Source: three-view drawing plus pictorial views. Frame: mm from the lowest corner of the part. A direction names the side the tool comes from. Give positions to 0.01 mm unless a question says otherwise; leave off trailing zeros. Loops run counter-clockwise (first coordinate to the right, second up) from the corner with the lowest first, then second, coordinate; pieces in that order, holes last. Notation, with made-up numbers: (89, 76) - (122, 76) arc R17 ccw to (122, 108) - close; hole circle Ø9 at (8, 51.25). An arc over 180 degrees is marked (long way). Put each result on its own line as item: value.
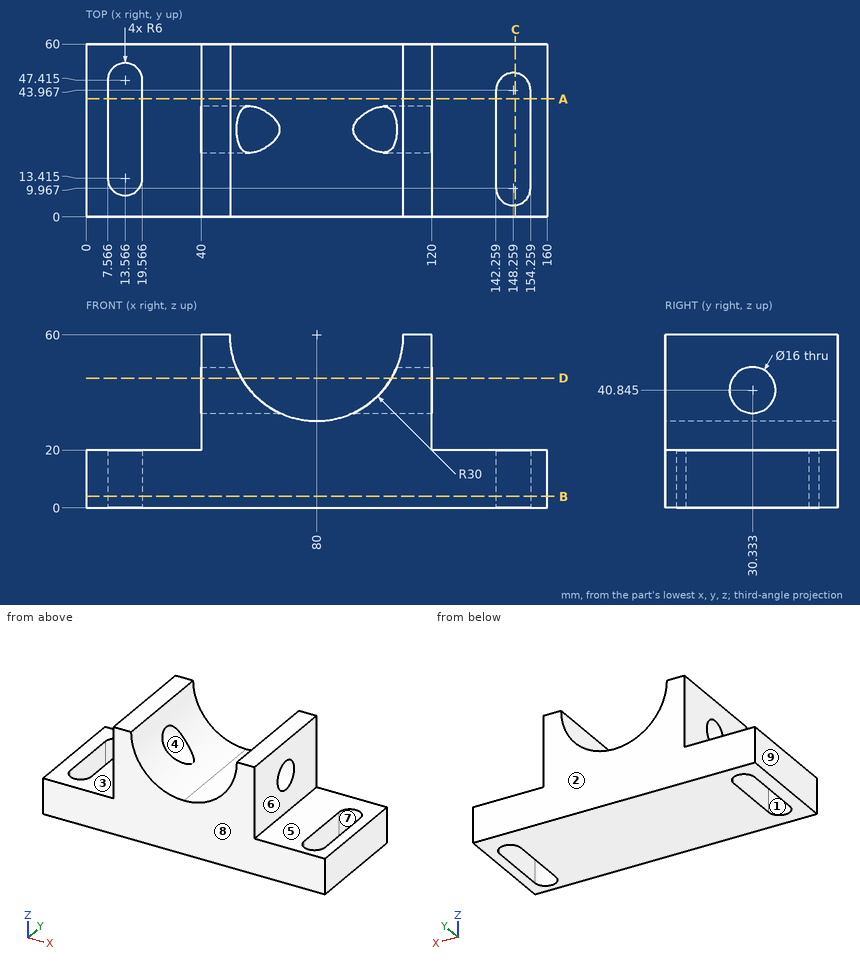
1) Section query C-C, the plane x = 149. Output: boundary loops of the cut face in (y, z), plus the area to 3 significant figures.
Check result:
outline: (0, 0) - (4.01, 0) - (4.01, 20) - (0, 20) - close; (49.92, 0) - (60, 0) - (60, 20) - (49.92, 20) - close
area: 282 mm²
2) Section query D-D, the plane z = 45. Output: boundary loops of the cut face in (x, y).
Check result:
outline: (40, 0) - (54.02, 0) - (54.02, 23.5) - (40, 23.5) - close; (40, 37.17) - (54.02, 37.17) - (54.02, 60) - (40, 60) - close; (105.98, 0) - (120, 0) - (120, 23.5) - (105.98, 23.5) - close; (105.98, 37.17) - (120, 37.17) - (120, 60) - (105.98, 60) - close
3) Mould query, pull axis X, two halves, no side actions, for the marked faces 6, 7, 8 and 9. Classes: pulls with the +X half, pulls with the -X half, needs draft (parallel to the pull), parting line crosses it, or undercut.
Check result:
face 6: pulls with the +X half
face 7: undercut
face 8: needs draft
face 9: pulls with the -X half
4) Access query for the marked faces 1, 2, 3, 4 and 5. Directions: +Z, -Z, +X, -X, +Y, -Y. A direction counts if a zero-diameter tool reaches every point of the face in a straight line with its end or side. Return the directions, or none.
Check result:
face 1: +Z, -Z
face 2: +Z, -Z, +X, -X, +Y
face 3: +Z, -X, +Y, -Y
face 4: +X, -X
face 5: +Z, +X, +Y, -Y
5) Section query B-B, the plane z = 4. Output: boundary loops of the cut face in (x, y) (1 decimal).
Check result:
outline: (0, 0) - (160, 0) - (160, 60) - (0, 60) - close; hole (7.6, 13.4) arc R6 ccw to (19.6, 13.4) - (19.6, 47.4) arc R6 ccw to (7.6, 47.4) - close; hole (142.3, 10) arc R6 ccw to (154.3, 10) - (154.3, 44) arc R6 ccw to (142.3, 44) - close
6) Section query A-A, the plane y = 41. Output: boundary loops of the cut face in (x, z), plus the area to 3 significant figures.
Check result:
outline: (0, 0) - (7.57, 0) - (7.57, 20) - (0, 20) - close; (19.57, 0) - (142.26, 0) - (142.26, 20) - (120, 20) - (120, 60) - (110, 60) arc R30 cw to (80, 30) arc R30 cw to (50, 60) - (40, 60) - (40, 20) - (19.57, 20) - close; (154.26, 0) - (160, 0) - (160, 20) - (154.26, 20) - close
area: 4,510 mm²
7) Pin query (flat end, axial travel): P1, Ø20, axis at y = 33.5, z = 36.5, coming from the +X side; P2, Ø1, axis at y = 44, z = 53.5, coming from the -X side; P3, Ø12, axis at x = 141, y = 17, coming from the +Z side. Return the tip coordinate at first contact, or that it passes through.
Check result:
P1: x = 120
P2: x = 40
P3: z = 20
8) Material intervals for line 1 along X through (y, z) = (35.5, 9.5); line 2 along X through (y, z) = (44.5, 9.5) (1 decimal); line 3 along Z through (x, y) = (79, 20), sorted ascending. Write a range as [from, to].
Check result:
line 1: [0, 7.57], [19.57, 142.26], [154.26, 160]
line 2: [0, 7.6], [19.6, 142.3], [154.2, 160]
line 3: [0, 30.02]
